from build123d import *

# Parameters (mm, degrees)
SKETCH1_W               = 49.35
SKETCH1_H               = 24.55
BOSS_EXTRUDE1_DEPTH     = 2
BOSS_EXTRUDE2_DEPTH     = 6.25
BOSS_EXTRUDE3_START     = -2
BOSS_EXTRUDE3_DEPTH     = 8.25
CUT_EXTRUDE1_DEPTH      = 33.889873061
CUT_EXTRUDE1_DEPTH_BACK = 33.889873061
SKETCH3_R               = 8.25
SKETCH3_R_2             = 1.825


with BuildPart() as part:
    # Sketch1 → Boss-Extrude1 (new body)
    with BuildSketch(Plane(origin=(0, 0, 0), x_dir=(1, 0, 0), z_dir=(0, 1, 0))):
        Rectangle(SKETCH1_W, SKETCH1_H)
    extrude(amount=BOSS_EXTRUDE1_DEPTH)

    # Sketch2 → Boss-Extrude2 (add)
    with BuildSketch(Plane(origin=(0, 2, 0), x_dir=(1, 0, 0), z_dir=(0, 1, 0))):
        Polygon((-24.675, 12.275), (-24.675, -12.275), (24.675, -12.275), (24.675, 12.275), (5.125, 12.275), (5.125, 10.525), (22.925, 10.525), (22.925, -10.525), (-22.925, -10.525), (-22.925, 10.525), (-5.125, 10.525), (-5.125, 12.275), align=None)
    extrude(amount=BOSS_EXTRUDE2_DEPTH)

    # Sketch4 → Boss-Extrude3 (add)
    with BuildSketch(Plane(origin=(0, 2, 0), x_dir=(1, 0, 0), z_dir=(0, 1, 0)).offset(BOSS_EXTRUDE3_START)):
        with BuildLine():
            Line((-24.675, 12.275), (-24.675, 8.775))
            ThreePointArc((-24.675, 8.775), (-27.149873734, 14.749873734), (-21.175, 12.275))
            Line((-21.175, 12.275), (-24.675, 12.275))
        make_face()
        with BuildLine():
            Line((-24.675, -12.275), (-24.675, -8.775))
            ThreePointArc((-24.675, -8.775), (-27.149873734, -14.749873734), (-21.175, -12.275))
            Line((-21.175, -12.275), (-24.675, -12.275))
        make_face()
        with BuildLine():
            Line((24.675, -12.275), (21.175, -12.275))
            ThreePointArc((21.175, -12.275), (27.149873734, -14.749873734), (24.675, -8.775))
            Line((24.675, -8.775), (24.675, -12.275))
        make_face()
        with BuildLine():
            Line((24.675, 8.775), (24.675, 12.275))
            Line((24.675, 12.275), (21.175, 12.275))
            ThreePointArc((21.175, 12.275), (27.149873734, 14.749873734), (24.675, 8.775))
        make_face()
    extrude(amount=BOSS_EXTRUDE3_DEPTH)

    # Sketch3 → Cut-Extrude1 (cut, two sides: drawn at the far end of the back side and taken through both)
    with BuildSketch(Plane(origin=(0, 2, 0), x_dir=(1, 0, 0), z_dir=(0, 1, 0)).offset(-CUT_EXTRUDE1_DEPTH_BACK)):
        with Locations(Location((-13.025, 0, 0), (0, 0, 270))):
            Circle(SKETCH3_R)
        with Locations(Location((13.025, 0, 0), (0, 0, 270))):
            Circle(SKETCH3_R)
        with Locations(Location((-24.675, 12.275, 0), (0, 0, 270))):
            Circle(SKETCH3_R_2)
        with Locations(Location((-24.675, -12.275, 0), (0, 0, 270))):
            Circle(SKETCH3_R_2)
        with Locations(Location((24.675, 12.275, 0), (0, 0, 270))):
            Circle(SKETCH3_R_2)
        with Locations(Location((24.675, -12.275, 0), (0, 0, 270))):
            Circle(SKETCH3_R_2)
        with BuildLine():
            Line((-3, -4.975), (3.25, -4.975))
            ThreePointArc((3.25, -4.975), (5.625, -7.35), (3.25, -9.725))
            Line((3.25, -9.725), (-3, -9.725))
            ThreePointArc((-3, -9.725), (-5.375, -7.35), (-3, -4.975))
        make_face()
    extrude(amount=CUT_EXTRUDE1_DEPTH + CUT_EXTRUDE1_DEPTH_BACK, mode=Mode.SUBTRACT)


solid = part.part
For this review, take the finished solid that the model builds, in its own axes (mm). A direction names the side the tool comes from. Coordinates: 2 decimals unless noted, no trailing zeros. Write each loop counter-clockwise with the first axis right and the second up, starting at its lowest first coordinate (ties: lowest second). Pieces come first, ordered by that corner, then holes. Notation, with made-up numbers: (-6, 60) -> (17, 60) arc R5 ccw to (17, 67) -> close; hole circle Ø4 at (4.5, 18.25). An arc over 180 degrees is marked (long way). Write each question's results on one line, items separated by ' | '. Start each with the question number.
1) Wall thickness on L1, parallel to X at y = 1.55, z = 0 (3 decimals); L2, parallel to X at y = 3.5, z = 8.5 (3 decimals); L3, parallel to Z at x = -8, y = 3 (3 decimals): over which ranges is each line inside the solid? List them lowest first. Write a range as [from, to].
2) Consider section D-D (z = -7.5). Write out the cut boundary in (x, y) (3 decimals), plus the area to 3 significant figures.
3) Consider section B-B (y = 4.25). Write out the cut boundary in (x, z) (3 decimals), plus the area to 3 significant figures.
4) Insertion check: pin 1 (3 mm diameter, centred on y = 4.5, z = -3.5, fed in from +X) (3 decimals); pin 2 (1.9 mm diameter, centred on x = 12, y = 4, fed in from +Z) (3 decimals); pin 3 (3 mm diameter, centred on x = 7.5, y = 5.5, fed in from -Z) (3 decimals); pin 4 (2 mm diameter, centred on x = -24.675, z = -12.275, fed in from -Y). Each pin has a flat end and moves straight along its axis. Give the tip position at first contact, or say it passes through.
5) For faces 1 (the face through (-24.675, 4, 0)), 2 (the face through (24.675, 4, 0)), 3 (the face through (0, 1, 4.975)), 4 (the face through (14, 5, -10.525)), 5 (the face through (5.125, 5, -11)), list the 3-axis set-ups (+Z, -Z, +X, -X, +Y, -Y) from which the entire face can be reached by the end or side of a thin tool; tool diameter is ignored.
6) Consider section C-C (z = 7.35). Write out the cut boundary in (x, y) (3 decimals), plus the area to 3 significant figures.
7) The part is to be moulded in two halves that separate along Z. For faces 6 (the face through (0, 1, -12.275)), 7 (the face through (0, 4, 12.275)), 8 (the face through (5.624, 0.986, 7.298)), say which applies: +Z half, -Z half, draft (parallel to the pull), parting line (faces both ways), or undercut.
8) Consider section A-A (x = 18). Write out the cut boundary in (y, z) (3 decimals), plus the area to 3 significant figures.
Geometry says:
1) L1: [-24.675, -21.275], [-4.775, 4.775], [21.275, 24.675] | L2: [-24.675, -22.925], [22.925, 24.675] | L3: [-12.275, -10.525], [10.525, 12.275]
2) outline: (-24.675, 0) -> (-16.462, 0) -> (-16.462, 2) -> (-22.925, 2) -> (-22.925, 8.25) -> (-24.675, 8.25) -> close; (-9.588, 0) -> (9.588, 0) -> (9.588, 2) -> (-9.588, 2) -> close; (16.462, 0) -> (24.675, 0) -> (24.675, 8.25) -> (22.925, 8.25) -> (22.925, 2) -> (16.462, 2) -> close | area: 93.1 mm^2
3) outline: (-24.675, -8.775) arc R3.5 ccw (long way) to (-21.175, -12.275) -> (-5.125, -12.275) -> (-5.125, -10.525) -> (-22.925, -10.525) -> (-22.925, 10.525) -> (22.925, 10.525) -> (22.925, -10.525) -> (5.125, -10.525) -> (5.125, -12.275) -> (21.175, -12.275) arc R3.5 ccw (long way) to (24.675, -8.775) -> (24.675, 8.775) arc R3.5 ccw (long way) to (21.175, 12.275) -> (-21.175, 12.275) arc R3.5 ccw (long way) to (-24.675, 8.775) -> close; hole circle Ø3.65 at (-24.675, -12.275); hole circle Ø3.65 at (-24.675, 12.275); hole circle Ø3.65 at (24.675, -12.275); hole circle Ø3.65 at (24.675, 12.275) | area: 302 mm^2
4) pin 1: x = 24.675 | pin 2: z = 12.275 | pin 3: z = -12.275 | pin 4: through
5) face 1: -X, +Y, -Y | face 2: +X, +Y, -Y | face 3: +Y, -Y | face 4: +Y | face 5: -Z, +Y
6) outline: (-24.675, 0) -> (-16.772, 0) -> (-16.772, 2) -> (-22.925, 2) -> (-22.925, 8.25) -> (-24.675, 8.25) -> close; (-9.278, 0) -> (-5.375, 0) -> (-5.375, 2) -> (-9.278, 2) -> close; (5.625, 0) -> (9.278, 0) -> (9.278, 2) -> (5.625, 2) -> close; (16.772, 0) -> (24.675, 0) -> (24.675, 8.25) -> (22.925, 8.25) -> (22.925, 2) -> (16.772, 2) -> close | area: 68.6 mm^2
7) face 6: -Z half | face 7: +Z half | face 8: undercut
8) outline: (0, -12.275) -> (8.25, -12.275) -> (8.25, -10.525) -> (2, -10.525) -> (2, -6.581) -> (0, -6.581) -> close; (0, 6.581) -> (2, 6.581) -> (2, 10.525) -> (8.25, 10.525) -> (8.25, 12.275) -> (0, 12.275) -> close | area: 44.7 mm^2
